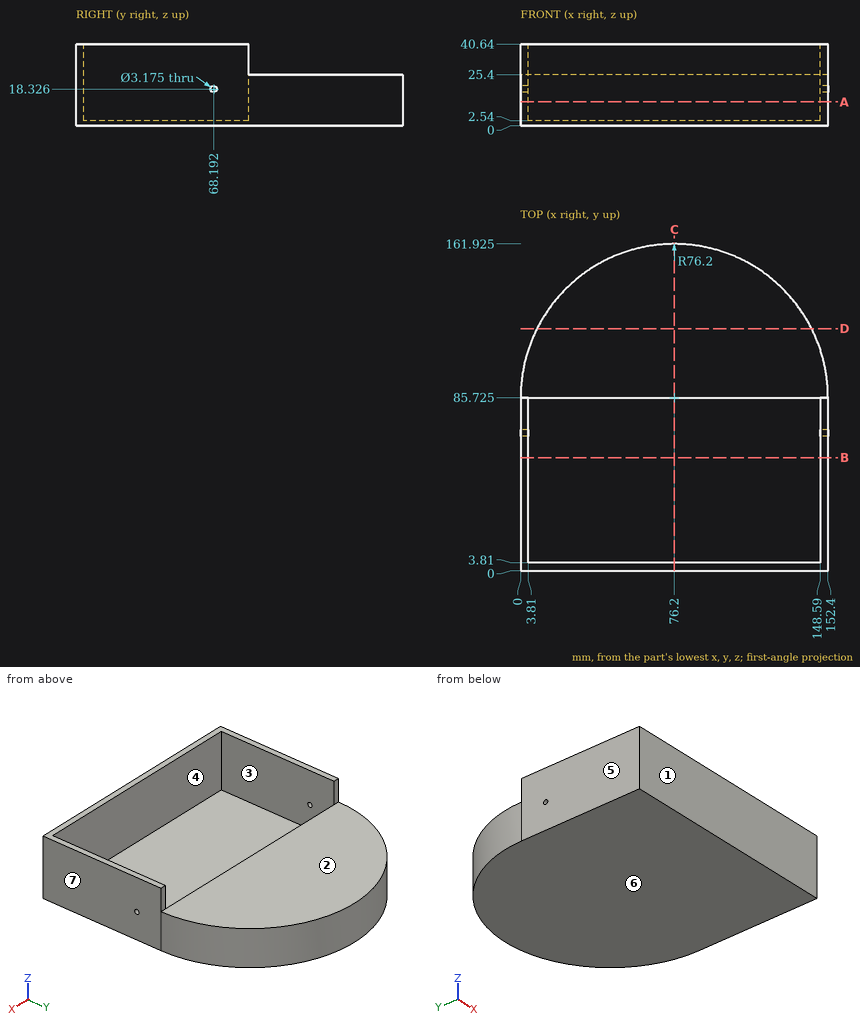
Geometry: see drawing. Coordinates: mm, zero at the bounding-box minimum. A direction names the side the tool comes from. Give positions to 0.01 mm unless a question says otherwise; leave off trailing zeros. Write each loop counter-clockwise with the first axis right and the second up, starting at its lowest first coordinate (ties: lowest second). Pieces come first, ordered by that corner, then holes. Notation, with made-up numbers: (76, 37.25) -> (132, 37.25) arc R33 cw to (132, 73.25) -> close; hole circle Ø1 at (30, 50). An arc over 180 degrees is marked (long way). Use one line per item in the form item = value. Start each with the question number.
1) Ray query, probe 1 along X at (y, z) = (42, 31); probe 2 along Y at (x, z) = (130.5, 6) (1 decimal); probe 3 along Y at (x, z) = (103, 12) (1 decimal). Return the intervals inside material, ascending. Write a range as from..to.
2) Section query B-B on y = 56. Return the cut outline in (x, z).
3) Section query C-C on x = 76.2. Return the cut outline in (y, z) (1 decimal).
4) Draft query along X for the marked faces 4, 5, 6 and 7. Return one class per face: pulls with the +X half, pulls with the -X half, needs draft (parallel to the pull), parting line crosses it, or undercut.
5) Set-up query: the marked faces 1, 2 and 3. Return all of +Z, -Z, +X, -X, +Y, -Y with unobstructed straight access to the full face (end or side cutting, diameter ignored); none if empty.
6) Section query D-D on y = 120. Return the cut outline in (x, z).
7) Pin query (flat end, axial travel): pin 1 (5 mm diameter, centred on x = 137, y = 39, fed in from +Z); pin 2 (4 mm diameter, centred on x = 151, z = 35.5, fed in from +Y) (3 decimals); pin 3 (1.5 mm diameter, centred on x = 120, z = 21.5, fed in from +Y). Return the tip coordinate at first contact, or that it passes through.
8) Section query A-A on z = 12. Return the cut outline in (x, y) (1 decimal), then the cut area to 3 significant figures.
Outcome:
q1.probe_1 = 0..3.81, 148.59..152.4
q1.probe_2 = 0..3.8, 85.7..139.2
q1.probe_3 = 0..3.8, 85.7..157.1
q2.outline = (0, 0) -> (152.4, 0) -> (152.4, 40.64) -> (148.59, 40.64) -> (148.59, 2.54) -> (3.81, 2.54) -> (3.81, 40.64) -> (0, 40.64) -> close
q3.outline = (0, 0) -> (161.9, 0) -> (161.9, 25.4) -> (85.7, 25.4) -> (85.7, 2.5) -> (3.8, 2.5) -> (3.8, 40.6) -> (0, 40.6) -> close
q4.face_4 = undercut
q4.face_5 = pulls with the -X half
q4.face_6 = needs draft
q4.face_7 = pulls with the +X half
q5.face_1 = +Z, -Z, +X, -X, -Y
q5.face_2 = +Z, +X, -X, +Y
q5.face_3 = +Z
q6.outline = (8.14, 0) -> (144.26, 0) -> (144.26, 25.4) -> (8.14, 25.4) -> close
q7.pin_1 = 2.54
q7.pin_2 = 85.725
q7.pin_3 = 148.6
q8.outline = (0, 0) -> (152.4, 0) -> (152.4, 85.7) arc R76.2 ccw to (0, 85.7) -> close; hole (3.8, 3.8) -> (148.6, 3.8) -> (148.6, 85.7) -> (3.8, 85.7) -> close
q8.area = 10,300 mm^2
